Check sheet for the modelled part. Datum: model origin and axes. Units: mm. Face numbers are marked on the shaded views. A direction names the side the tool comes from. Round coordinates to 2 decimals unless told otherwise and drop trailing zeros. Loops run counter-clockwise (first coordinate to the right, second up) from the corner with the lowest first, then second, coordinate; pieces in that order, holes last. Notation, with made-up numbers: (-13, 13) - (-6, 13) arc R23 cw to (-6, 36) - close; hole circle Ø8 at (20, 46.25). An arc over 180 degrees is marked (long way). Return JSON: item names as keys, results as strings.
from build123d import *

# Parameters (mm, degrees)
F1_DEPTH = 50
F2_R     = 5
F3_R     = 6.5
F3_R_2   = 1.4
F4_DEPTH = 3.3
F5_DEPTH = 13.3
F6_R     = 3


with BuildPart() as f1:
    # F0 (on Front) → F1 (new body)
    with BuildSketch(Plane.XZ):
        Polygon((-50, 15), (-50, 0), (0, 0), (0, 50), (-10, 50), (-10, 15), align=None)
    extrude(amount=F1_DEPTH)

    # F2
    f2_edges = [f1.edges().sort_by_distance(p)[0] for p in [
        (-5, -50, 50),
        (-5, 0, 50),
    ]]
    fillet(f2_edges, radius=F2_R)

    # F3 (on face) → F4 (cut)
    with BuildSketch(Plane(origin=(-50, 0, 0), x_dir=(0, -1, 0), z_dir=(-1, 0, 0))):
        with Locations((8, 7.5)):
            Circle(F3_R)
        with Locations((8, 7.5)):
            Circle(F3_R_2, mode=Mode.SUBTRACT)
        with Locations((25, 7.5)):
            Circle(F3_R)
        with Locations((25, 7.5)):
            Circle(F3_R_2, mode=Mode.SUBTRACT)
        with Locations((42, 7.5)):
            Circle(F3_R)
        with Locations((42, 7.5)):
            Circle(F3_R_2, mode=Mode.SUBTRACT)
        with Locations((8, 7.5)):
            Circle(F3_R_2)
        with Locations((25, 7.5)):
            Circle(F3_R_2)
        with Locations((42, 7.5)):
            Circle(F3_R_2)
    extrude(amount=-F4_DEPTH, mode=Mode.SUBTRACT)

    # F3 (on face) → F5 (cut)
    with BuildSketch(Plane(origin=(-50, 0, 0), x_dir=(0, -1, 0), z_dir=(-1, 0, 0))):
        with Locations((8, 7.5)):
            Circle(F3_R_2)
        with Locations((25, 7.5)):
            Circle(F3_R_2)
        with Locations((42, 7.5)):
            Circle(F3_R_2)
    extrude(amount=-F5_DEPTH, mode=Mode.SUBTRACT)

    # F6
    f6_edges = [f1.edges().sort_by_distance(p)[0] for p in [
        (-25, -50, 0),
        (-25, 0, 0),
        (-30, 0, 15),
        (-30, -50, 15),
    ]]
    fillet(f6_edges, radius=F6_R)


solid = f1.part
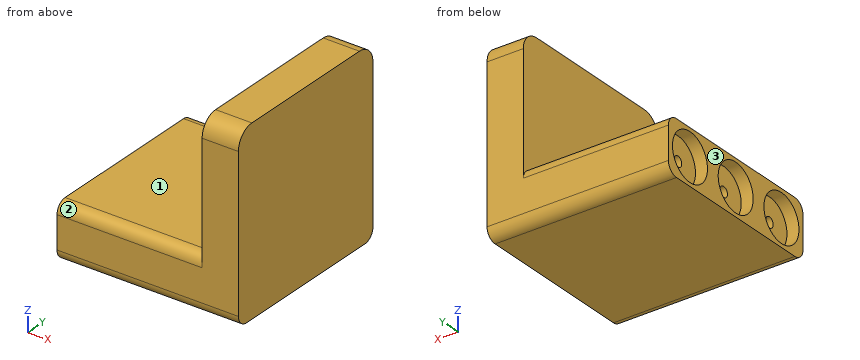
Q1. Scan lines: probe 1 along Z at (x, y) = (-39.5, -42); probe 2 along Y at (x, z) = (-48, 11.5); probe 3 along Z at (x, y) = (-48.75, -25). Record each from-to range of solid material in increasing order. Write a range as [from, to].
Answer key:
{"probe 1": "z = [0, 6.1], [8.9, 15]", "probe 2": "y = [-50, -47.12], [-36.88, -30.12], [-19.88, -13.12], [-2.88, 0]", "probe 3": "z = [0, 1], [14, 15]"}
Q2. Sectioned sample at A-A (x = -41). Enter the section's corners in (y, z), plus the area to 3 significant figures.
Answer key:
{"outline": "(-50, 3) arc R3 ccw to (-47, 0) - (-3, 0) arc R3 ccw to (0, 3) - (0, 12) arc R3 ccw to (-3, 15) - (-47, 15) arc R3 ccw to (-50, 12) - close; hole circle Ø2.8 at (-42, 7.5); hole circle Ø2.8 at (-25, 7.5); hole circle Ø2.8 at (-8, 7.5)", "area": "724 mm²"}
Q3. Tool access check on the marked faces 1, 2 and 3. Record the directions out of +Z, -Z, +X, -X, +Y, -Y that give a thin tool (end or side, any length) a straight path to the whole face; none if there is none.
Answer key:
{"face 1": "+Z, -X, +Y, -Y", "face 2": "+Z, -X, -Y", "face 3": "+Z, -Z, -X, +Y, -Y"}
Q4. Depth check by flat-ended pin: P1, Ø6.5, axis at y = -23.5, z = 7.5, coming from the -X side; P2, Ø3, axis at x = -29, y = -27, coming from the +Z side; P3, Ø0.8, axis at y = -8, z = 7, coming from the -X side. Enter the tip coordinate at first touch or a pass-through.
Answer key:
{"P1": "stops at x = -46.7", "P2": "stops at z = 15", "P3": "stops at x = -36.7"}
Q5. Sectioned sample at B-B (y = -8). Enter the section's corners in (x, z).
Answer key:
{"outline": "(-50, 0) - (0, 0) - (0, 50) - (-10, 50) - (-10, 15) - (-50, 15) - (-50, 14) - (-46.7, 14) - (-46.7, 8.9) - (-36.7, 8.9) - (-36.7, 6.1) - (-46.7, 6.1) - (-46.7, 1) - (-50, 1) - close"}
Q6. Sectioned sample at D-D (z = 34). Enter the section's corners in (x, y).
Answer key:
{"outline": "(-10, -50) - (0, -50) - (0, 0) - (-10, 0) - close"}
Q7. Sectioned sample at C-C (x = -34). Enter the section's corners in (y, z), plus the area to 3 significant figures.
Answer key:
{"outline": "(-50, 3) arc R3 ccw to (-47, 0) - (-3, 0) arc R3 ccw to (0, 3) - (0, 12) arc R3 ccw to (-3, 15) - (-47, 15) arc R3 ccw to (-50, 12) - close", "area": "742 mm²"}
